```python
from build123d import *

# Parameters (mm, degrees)
F1_DEPTH = 279.4
F2_W     = 57.15
F2_H     = 88.9
F3_DEPTH = 5.5636
F6_D     = 4.7625
F7_D     = 3.175
F9_D     = 6.35


with BuildPart() as f1:
    # F0 (on Right) → F1 (new body)
    with BuildSketch(Plane.YZ):
        with BuildLine():
            Line((0, 5.5626), (0, 0))
            Line((0, 0), (67.0687, 0))
            ThreePointArc((67.0687, 0), (73.525504, 2.674496), (76.2, 9.1313))
            Line((76.2, 9.1313), (76.2, 349.25))
            Line((76.2, 349.25), (70.6374, 349.25))
            Line((70.6374, 349.25), (70.6374, 9.1313))
            ThreePointArc((70.6374, 9.1313), (69.592152, 6.607848), (67.0687, 5.5626))
            Line((67.0687, 5.5626), (0, 5.5626))
        make_face()
    extrude(amount=F1_DEPTH)

    # F2 (on face) → F3 (cut, through all)
    with BuildSketch(Plane.XZ.offset(-70.6374)):
        with Locations((250.825, 304.8)):
            Rectangle(F2_W, F2_H)
    extrude(amount=-F3_DEPTH, mode=Mode.SUBTRACT)

    # F6 (through all)
    with Locations(Plane(origin=(0, 76.2, 0), x_dir=(-1, 0, 0), z_dir=(0, 1, 0))):
        with Locations((-187.325, 342.9), (-187.325, 279.4), (-187.325, 215.9), (-187.325, 152.4), (-187.325, 88.9), (-165.1, 25.4), (-165.1, 88.9), (-165.1, 152.4), (-165.1, 215.9), (-165.1, 279.4), (-111.125, 342.9), (-111.125, 279.4), (-111.125, 215.9), (-111.125, 152.4), (-111.125, 88.9), (-88.9, 25.4), (-88.9, 88.9), (-88.9, 152.4), (-88.9, 215.9), (-88.9, 279.4), (-22.225, 314.325)):
            Hole(F6_D / 2)

    # F7 (through all)
    with Locations(Plane(origin=(0, 76.2, 0), x_dir=(-1, 0, 0), z_dir=(0, 1, 0))):
        with Locations((-261.183679, 137.900822), (-221.508879, 116.463222), (-221.508879, 143.489555), (-260.35, 164.927155), (-260.35, 192.092642), (-220.6752, 170.655042), (-220.6752, 198.442642), (-260.35, 227.75419)):
            Hole(F7_D / 2)

    # F9 (through all)
    with Locations(Plane(origin=(0, 0, 0), x_dir=(1, 0, 0), z_dir=(0, 0, -1))):
        with Locations((88.9, -12.7), (190.5, -12.7)):
            Hole(F9_D / 2)


solid = f1.part
```
Build history of the part. All positions in model axes, mm. A direction names the side the tool comes from. Coordinates: 2 decimals unless noted, no trailing zeros. Order: outer loops, then holes, each group sorted by start corner. A loop starts at its lowest first (then second) coordinate and runs counter-clockwise, first axis right, second up. Notation, with made-up numbers: M 7.5,41 L 25.5,41 A19 cw 25.5,61 Z; hole C -28.75,66.25 d3. An arc over 180 degrees is marked long. One line per question, with ' | ' between items. Start each with the question number.
1. Cut at C-C (z = 129). Write the cut outline in (x, y).
2. Flat gauge pins, fed straight in: P1, Ø4, axis at x = 220.68, z = 170.66, coming from the -Y side; P2, Ø1.7, axis at y = 74, z = 311, coming from the +X side; P3, Ø4.5, axis at x = 165.1, z = 215.9, coming from the +Y side; P4, Ø5, axis at x = 220.5, y = 45.5, coming from the +Z side. Where does each tip first touch, or does it go through?
3. Tool access for faces 1 (the face through (0, 72, 175)), 2 (the face through (138, 34, 5.563)): list every direction of +Z, -Z, +X, -X, +Y, -Y with a clear straight run to the whole face (end or side of a thin tool).
4. Cut at A-A (x = 212.5). Write the cut outline in (y, z).
5. Wall check: line 1 along X through (y, z) = (74.45, 279.4); line 2 along X through (y, z) = (73.6, 152.4); line 3 along X through (y, z) = (12.7, 1.6) (3 decimals). Give the ranges that are in metal, low to high. Write a range as [from, to].
6. Cut at B-B (y = 49). Write the cut outline in (x, z), plus the area to 3 significant figures.
The answers:
1) outline: M 0,70.64 L 279.4,70.64 L 279.4,76.2 L 0,76.2 Z
2) P1: stops at y = 70.64 | P2: stops at x = 222.25 | P3: passes through | P4: stops at z = 5.56
3) face 1: +Z, -Z, -X, +Y, -Y | face 2: +Z, +X, -X, -Y
4) outline: M 0,0 L 67.07,0 A9.13 ccw 76.2,9.13 L 76.2,349.25 L 70.64,349.25 L 70.64,9.13 A3.57 cw 67.07,5.56 L 0,5.56 Z
5) line 1: x = [0, 86.52], [91.28, 108.74], [113.51, 162.72], [167.48, 184.94], [189.71, 222.25] | line 2: x = [0, 86.52], [91.28, 108.74], [113.51, 162.72], [167.48, 184.94], [189.71, 279.4] | line 3: x = [0, 85.725], [92.075, 187.325], [193.675, 279.4]
6) outline: M 0,0 L 279.4,0 L 279.4,5.56 L 0,5.56 Z | area: 1,550 mm2
